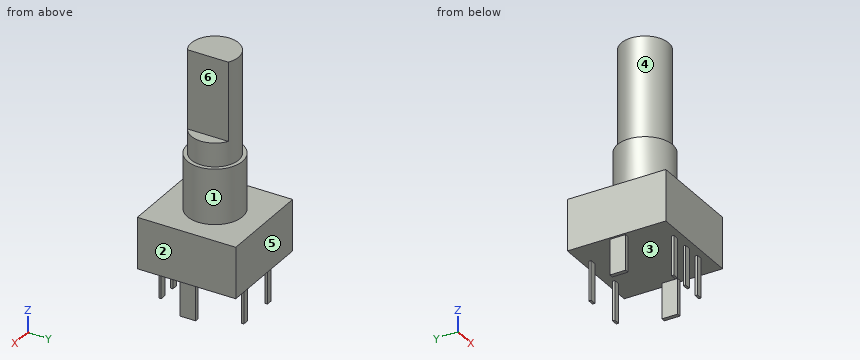
```python
from build123d import *

# Parameters (mm, degrees)
SKETCH1_W     = 12
SKETCH1_H     = 12.5
BODY_DEPTH    = 6.5
SKETCH2_R     = 3.5
BUSHING_DEPTH = 7
SKETCH3_R     = 3
SHAFT_DEPTH   = 13
SKETCH4_W     = 0.8
SKETCH4_H     = 0.3
PINS_DEPTH    = 5
SKETCH5_W     = 0.5
SKETCH5_H     = 2
TABS_DEPTH    = 4.5
SKETCH6_W     = 4
SKETCH6_H     = 8
D_FLAT_DEPTH  = 10


with BuildPart() as part:
    # Sketch1 → Body (new body)
    with BuildSketch(Plane.XY):
        Rectangle(SKETCH1_W, SKETCH1_H)
    extrude(amount=BODY_DEPTH)

    # Sketch2 → Bushing (add)
    with BuildSketch(Plane.XY.offset(6.5)):
        Circle(SKETCH2_R)
    extrude(amount=BUSHING_DEPTH)

    # Sketch3 → Shaft (add)
    with BuildSketch(Plane.XY.offset(13.5)):
        Circle(SKETCH3_R)
    extrude(amount=SHAFT_DEPTH)

    # Sketch4 → Pins (add)
    with BuildSketch(Plane.XY):
        with Locations((-2.5, -5.25)):
            Rectangle(SKETCH4_W, SKETCH4_H)
        with Locations((0, -5.25)):
            Rectangle(SKETCH4_W, SKETCH4_H)
        with Locations((2.5, -5.25)):
            Rectangle(SKETCH4_W, SKETCH4_H)
        with Locations((-2.5, 5.25)):
            Rectangle(SKETCH4_W, SKETCH4_H)
        with Locations((2.5, 5.25)):
            Rectangle(SKETCH4_W, SKETCH4_H)
    extrude(amount=-PINS_DEPTH)

    # Sketch5 → Tabs (add)
    with BuildSketch(Plane.XY):
        with Locations((-5.5, 0)):
            Rectangle(SKETCH5_W, SKETCH5_H)
        with Locations((5.5, 0)):
            Rectangle(SKETCH5_W, SKETCH5_H)
    extrude(amount=-TABS_DEPTH)

    # Sketch6 → D_flat (cut)
    with BuildSketch(Plane.XY.offset(26.5)):
        with Locations((3.5, 0)):
            Rectangle(SKETCH6_W, SKETCH6_H)
    extrude(amount=-D_FLAT_DEPTH, mode=Mode.SUBTRACT)


solid = part.part
```
Input: part model. Units: mm. Frame: model coordinates. Face numbers are marked on the shaded views. A direction names the side the tool comes from. Round coordinates to 2 decimals unless told otherwise and drop trailing zeros. Loops run counter-clockwise (first coordinate to the right, second up) from the corner with the lowest first, then second, coordinate; pieces in that order, holes last. Notation, with made-up numbers: (2, 41) -> (61, 41) arc R20 ccw to (61, 65) -> close; hole circle Ø2 at (29, 9.25). An arc over 180 degrees is marked (long way). Write each question's results on one line, items separated by ' | '.
1. Mould query, pull axis Y, two halves, no side actions, for the marked faces 1, 2 and 3. Classes: +Y half, -Y half, draft (parallel to the pull), parting line (faces both ways), or undercut.
Geometry results:
face 1: parting line | face 2: draft | face 3: undercut
2. Set-up query: the marked faces 4, 5 and 6. Return all of +Z, -Z, +X, -X, +Y, -Y with unobstructed straight access to the full face (end or side cutting, diameter ignored); none if empty.
Geometry results:
face 4: +Z | face 5: +Z, -Z, +X, -X, +Y | face 6: +Z, +X, +Y, -Y
3. Ray query, line 1 (Z direction, x = -3, y = 4); line 2 (Z direction, x = 2.5, y = -0.75); line 3 (Y direction, x = 0.75, z = 15.5). Return the intervals inside material, ascending. Write a range as from..to.
Geometry results:
line 1: 0..6.5 | line 2: 0..16.5 | line 3: -2.9..2.9
4. First-contact query: P1, Ø3, axis at x = 2.5, z = 22.5, coming from the +Y side; P2, Ø6, axis at x = 0, y = 0, coming from the -Z side; P3, Ø2, axis at x = -2, z = 17.5, coming from the -Y side. Flat tips, straight axial feed; report the tip coordinate or a pass-through.
Geometry results:
P1: y = 2.83 | P2: z = 0 | P3: y = -2.83
5. Section C-C (z = 20). Return loops of the section in (x, y), and give its area (3 significant figures).
Geometry results:
outline: (1.5, -2.6) -> (1.5, 2.6) arc R3 ccw (long way) to start | area: 22.7 mm2
6. Section D-D (z = 12). Return loops of the section in (x, y), and give its area (3 significant figures).
Geometry results:
outline: circle Ø7 at (0, 0) | area: 38.5 mm2
7. Section A-A (x = 0). Return loops of the section in (y, z).
Geometry results:
outline: (-6.25, 0) -> (-5.4, 0) -> (-5.4, -5) -> (-5.1, -5) -> (-5.1, 0) -> (6.25, 0) -> (6.25, 6.5) -> (3.5, 6.5) -> (3.5, 13.5) -> (3, 13.5) -> (3, 26.5) -> (-3, 26.5) -> (-3, 13.5) -> (-3.5, 13.5) -> (-3.5, 6.5) -> (-6.25, 6.5) -> close
8. Section B-B (y = 0). Return loops of the section in (x, z).
Geometry results:
outline: (-6, 0) -> (-5.75, 0) -> (-5.75, -4.5) -> (-5.25, -4.5) -> (-5.25, 0) -> (5.25, 0) -> (5.25, -4.5) -> (5.75, -4.5) -> (5.75, 0) -> (6, 0) -> (6, 6.5) -> (3.5, 6.5) -> (3.5, 13.5) -> (3, 13.5) -> (3, 16.5) -> (1.5, 16.5) -> (1.5, 26.5) -> (-3, 26.5) -> (-3, 13.5) -> (-3.5, 13.5) -> (-3.5, 6.5) -> (-6, 6.5) -> close
